Autodesk Inventor part; units mm, degrees
ref_plane "YZ Plane" through (0, 0, 0) normal (1, 0, 0) x (0, 1, 0)
ref_plane "XZ Plane" through (0, 0, 0) normal (0, 1, 0) x (-1, 0, 0)
ref_plane "XY Plane" through (0, 0, 0) normal (0, 0, 1) x (1, 0, 0)
sketch "Sketch1" plane through (0, 0, 0) normal (1, 0, 0) x (0, 1, 0)
  point P0 (0, 0)
sketch "Sketch2" plane through (0, 0, 0) normal (1, 0, 0) x (0, 1, 0)
  line L0 (-15.1188, 24.4143) -> (6.8812, 24.4143)
  line L1 (6.8812, 24.4143) -> (6.8812, -14.5857)
  line L2 (6.8812, -14.5857) -> (-15.1188, -14.5857)
  line L3 (-15.1188, -14.5857) -> (-15.1188, 24.4143)
  circle A0 centre (6.8812, 4.9143) radius 17.5
  point P0 (0, 0)
  point P1 (6.8812, -12.5857)
  point P2 (6.8812, 22.4143)
  dimension "d0" = 39
  dimension "d1" = 22
  dimension "d2" = 35
  dimension "d5" = 19.5
  dimension "d6" = 19.5
extrude "Extrusion1" add sketch "Sketch2" along normal blind 25 contours L0 L1 A0 L2 L3
sketch "Sketch3" plane through (25, 0, 0) normal (1, 0, 0) x (0, 0, -1)
  arc A0 (-22.4143, 6.8812) -> (12.5857, 6.8812) centre (-4.9143, 6.8812) ccw
  line L0 (-4.9143, 6.8812) -> (-7.9532, -10.3529)
  line L1 (-4.9143, 6.8812) -> (12.5857, 6.8812) construction
  line L2 (-7.9532, -10.3529) -> (-24.4143, -7.4504)
  line L3 (-24.4143, 6.8812) -> (-24.4143, -15.1188)
  line L4 (-24.4143, -7.4504) -> (-33.9046, 19.8743)
  line L5 (-33.9046, 19.8743) -> (-4.9143, 6.8812)
  point P0 (0, 0)
  dimension "d7" = 100
extrude "Extrusion2" cut sketch "Sketch3" against normal blind 37.625
properties part number "BaseArmHolder"
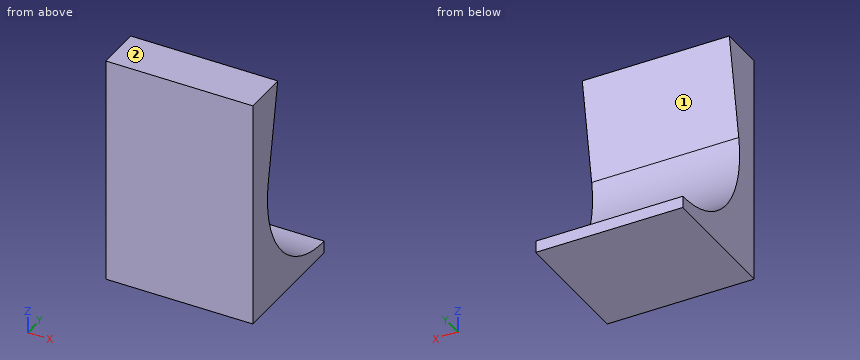
Read the model definition and answer for the solid it produces. Units are mm, in the model's axes. Face numbers are marked on the shaded views. A direction names the side the tool comes from. Round coordinates to 2 decimals unless told otherwise and drop trailing zeros. Write each loop counter-clockwise with the first axis right and the second up, starting at its lowest first coordinate (ties: lowest second). Pieces come first, ordered by that corner, then holes. Notation, with made-up numbers: (58, 62) -> (82, 62) arc R31 cw to (82, 86) -> close; hole circle Ø4 at (-18.5, 1). An arc over 180 degrees is marked (long way). Answer in a Markdown table with one row per item. Add a question column.
1) Find section A-A, the plane x = 22. Determine the outline of the cut face in (y, z).
2) Find section B-B, the plane z = 19. Determine the outline of the cut face in (x, y).
3) Given P1, Ø1.5, axis at x = 20.5, y = 4, coming from the +Z side; P2, Ø5, axis at x = 19, y = 1.5, coming from the +Z side; P3, Ø4, axis at x = 8.5, y = -2, coming from the +Z side, each flat-ended and moving along its own axis, determine where each tip first touches the part or whether it passes through.
4) Consider line 1 (Y direction, x = 13.75, z = 19.5); line 2 (Y direction, x = 16.25, z = 11.5); line 3 (Z direction, x = 21.5, y = -2). Determine where each line is inside the solid, lowest interval first.
5) Find section C-C, the plane y = 4.5. Determine the outline of the cut face in (x, z), and give its area (3 significant figures).
6) Which of the six approach directions +Z, -Z, +X, -X, +Y, -Y give full straight-line access (tool end or side, diameter ignored) to the marked faces 1 and 2?
Findings below:
| question | item | result |
|---|---|---|
| 1 | outline | (-15.12, -14.59) -> (6.88, -14.59) -> (6.88, -12.59) arc R17.5 cw to (-10.35, 7.95) -> (-7.45, 24.41) -> (-15.12, 24.41) -> close |
| 2 | outline | (0, -15.12) -> (25, -15.12) -> (25, -8.41) -> (0, -8.41) -> close |
| 3 | P1 | z = -12.2 |
| 3 | P2 | z = -10.71 |
| 3 | P3 | z = -8.79 |
| 4 | line 1 | -15.12 to -8.32 |
| 4 | line 2 | -15.12 to -9.73 |
| 4 | line 3 | -14.59 to -10.16 |
| 5 | outline | (0, -14.59) -> (25, -14.59) -> (25, -12.42) -> (0, -12.42) -> close |
| 5 | area | 54.1 mm² |
| 6 | face 1 | +X, -X, +Y |
| 6 | face 2 | +Z, +X, -X, +Y, -Y |
